Part model, mm, in its own coordinate system. Coordinates: 2 decimals unless noted, no trailing zeros. Loops run counter-clockwise (first coordinate to the right, second up) from the corner with the lowest first, then second, coordinate; pieces in that order, holes last. Notation, with made-up numbers: (48, 56) -> (76, 56) arc R21 ccw to (76, 92) -> close; hole circle Ø5 at (-31.5, 84). An arc over 180 degrees is marked (long way). One line per question, with ' | ' between items. Start each with the question number.
1) Drop flat-ended pins along their axis: pin 1 (0.8 mm diameter, centred on y = -1281.5, z = 2457.5, fed in from -X); pin 2 (3 mm diameter, centred on x = -1890, z = 2457.5, fed in from -Y); pin 3 (0.8 mm diameter, centred on x = -1894, z = 2458, fed in from +Y). Give the stop position or say it passes through.
2) Cut at B-B (y = -1266.5). List the corners of the cut face in (x, z).
3) Probe L1, parallel to Z at x = -1897.5, y = -1263; L2, parallel to X at y = -1276, z = 2457; L3, parallel to Z at x = -1903.5, y = -1271. List the from-to ranges inside material, lowest first. Write a range as from..to.
4) Cut at C-C (x = -1890). List the corners of the cut face in (y, z) (3 decimals).
5) Cut at D-D (y = -1285.5). List the corners of the cut face in (x, z), plus the area to 3 significant figures.
6) Cut at A-A (x = -1874.5). List the corners of the cut face in (y, z), plus the area to 3 significant figures.
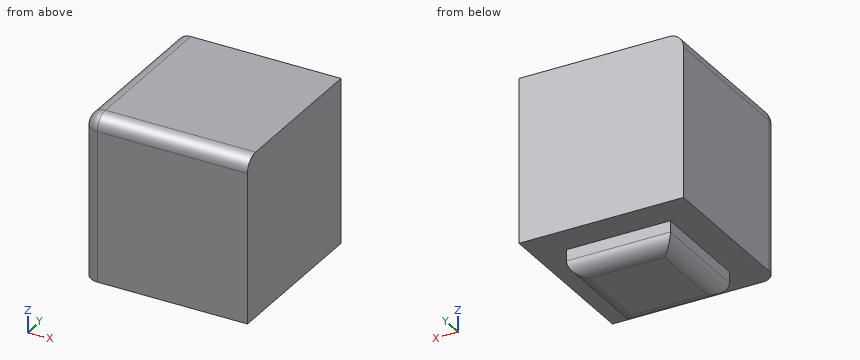
from build123d import *

# Parameters (mm, degrees)
SKETCH060_W             = 41.021
SKETCH060_H             = 41.021
PAD050_DEPTH            = 41.021
SKETCH059_W             = 25.908
SKETCH059_H             = 25.908
PAD049_DEPTH            = 6.35
FILLET005_R             = 3.556
FILLET004_R             = 3.556
BODY041_PLACEMENT_ANGLE = 270


with BuildPart() as part:
    # Sketch060 → Pad050 (new body)
    with BuildSketch(Plane.XZ):
        with Locations((20.5105, 20.5105)):
            Rectangle(SKETCH060_W, SKETCH060_H)
    extrude(amount=PAD050_DEPTH)

    # Sketch059 (on Face3 of Pad050) → Pad049 (join)
    with BuildSketch(Plane(origin=(0, 0, 0), x_dir=(1, 0, 0), z_dir=(0, 0, -1))):
        with Locations((20.507403, 20.507403)):
            Rectangle(SKETCH059_W, SKETCH059_H)
    extrude(amount=PAD049_DEPTH)

    # Fillet005
    fillet005_edges = [part.edges().sort_by_distance(p)[0] for p in [
        (7.553403, -20.507403, -6.35),
        (20.507403, -33.461403, -6.35),
        (20.507403, -7.553403, -6.35),
        (33.461403, -20.507403, -6.35),
    ]]
    fillet(fillet005_edges, radius=FILLET005_R)

    # Fillet004
    fillet004_edges = [part.edges().sort_by_distance(p)[0] for p in [
        (20.5105, -41.021, 41.021),
        (41.021, -41.021, 20.5105),
        (41.021, -20.5105, 41.021),
    ]]
    fillet(fillet004_edges, radius=FILLET004_R)


with BuildPart() as part_1:
    # Body041 placement: moved
    add(part.part.moved(Location((-1870.402819, -1260.805597, 2459.1772))).rotate(Axis((-1870.402819, -1260.805597, 2459.1772), (0, 0, 1)), BODY041_PLACEMENT_ANGLE))


solid = part_1.part
Reported:
1) pin 1: stops at x = -1903.86 | pin 2: stops at y = -1294.27 | pin 3: stops at y = -1268.36
2) outline: (-1911.42, 2459.18) -> (-1870.4, 2459.18) -> (-1870.4, 2500.2) -> (-1907.87, 2500.2) arc R3.56 ccw to (-1911.42, 2496.64) -> close
3) L1: z = 2459.18..2500.2 | L2: x = -1903.86..-1877.96 | L3: z = 2454.82..2500.2
4) outline: (-1301.827, 2459.177) -> (-1294.267, 2459.177) -> (-1294.267, 2456.383) arc R3.556 ccw to (-1290.711, 2452.827) -> (-1271.915, 2452.827) arc R3.556 ccw to (-1268.359, 2456.383) -> (-1268.359, 2459.177) -> (-1260.806, 2459.177) -> (-1260.806, 2500.198) -> (-1298.271, 2500.198) arc R3.556 ccw to (-1301.827, 2496.642) -> close
5) outline: (-1911.42, 2459.18) -> (-1903.86, 2459.18) -> (-1903.86, 2456.38) arc R3.56 ccw to (-1900.31, 2452.83) -> (-1881.51, 2452.83) arc R3.56 ccw to (-1877.96, 2456.38) -> (-1877.96, 2459.18) -> (-1870.4, 2459.18) -> (-1870.4, 2500.2) -> (-1907.87, 2500.2) arc R3.56 ccw to (-1911.42, 2496.64) -> close | area: 1,840 mm²
6) outline: (-1301.83, 2459.18) -> (-1260.81, 2459.18) -> (-1260.81, 2500.2) -> (-1298.27, 2500.2) arc R3.56 ccw to (-1301.83, 2496.64) -> close | area: 1,680 mm²
